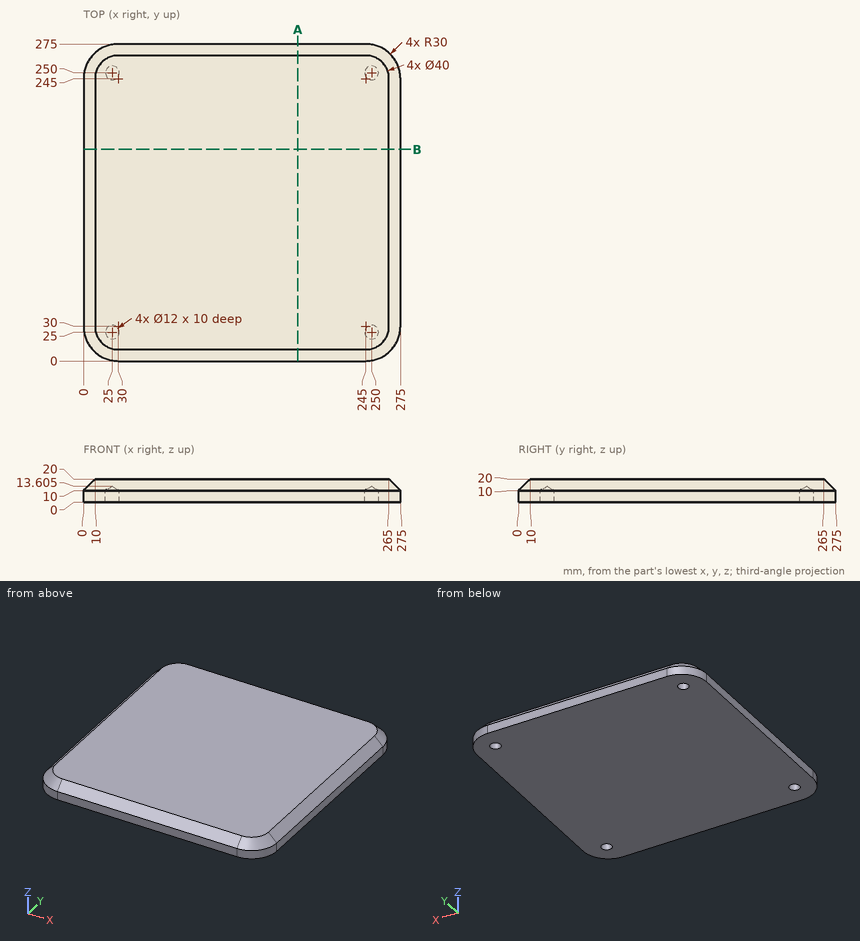
Print and shaded views of the part. All mm, measured from the part's lowest x, y and z. Round coordinates to 2 decimals unless told otherwise and drop trailing zeros. Loops run counter-clockwise (first coordinate to the right, second up) from the corner with the lowest first, then second, coordinate; pieces in that order, holes last. Notation, with made-up numbers: (13, 3.25) -> (69, 3.25) arc R18 ccw to (69, 17.25) -> close; hole circle Ø10 at (44.25, 20). An arc over 180 degrees is marked (long way). Use CSV: the item, a comma, the result in double quotes. Start each with the question number.
1) Cut at A-A, the plane x = 186. Write the cut outline in (y, z), plus the area to 3 significant figures.
2) Drop flat-ended pins along their axis: P1, Ø11, axis at x = 250, y = 25, coming from the -Z side; P2, Ø1, axis at x = 208.5, z = 16, coming from the +Y side; P3, Ø4, axis at x = 187, z = 16, coming from the +Y side. Give the stop position or say it passes through.
3) Wall check: L1, parallel to Y at x = 25, z = 6.25; L2, parallel to X at y = 197, z = 16. Give the ranges that are in metal, low to high. Write a range as [from, to].
Determined:
1,outline,"(0, 0) -> (275, 0) -> (275, 10) -> (265, 20) -> (10, 20) -> (0, 10) -> close"
1,area,"5,400 mm2"
2,P1,"stops at z = 10.3"
2,P2,"stops at y = 269.5"
2,P3,"stops at y = 271"
3,L1,"y = [0.42, 19], [31, 244], [256, 274.58]"
3,L2,"x = [6, 269]"
